For this review, take the finished solid that the model builds, in its own axes (mm). A direction names the side the tool comes from. Give positions to 0.01 mm unless a question says otherwise; leave off trailing zeros. Order: outer loops, then holes, each group sorted by start corner. A loop starts at its lowest first (then second) coordinate and runs counter-clockwise, first axis right, second up.
from build123d import *

# Parameters (mm, degrees)
CHAMFER1_SIZE = 1.25


with BuildPart() as part:
    # Sketch1 → Revolve1 (revolve)
    with BuildSketch(Plane(origin=(0, 0, 0), x_dir=(0, 0, -1), z_dir=(1, 0, 0))):
        with BuildLine():
            Line((0, 0), (0, 85.55))
            Line((0, 85.55), (3.18, 85.55))
            Line((3.18, 85.55), (3.18, 15.100044805))
            ThreePointArc((3.18, 15.100044805), (10.945145292, 4.426569715), (24.13, 3.81))
            Line((24.13, 3.81), (26.67, 1.27))
            Line((26.67, 1.27), (26.67, 0))
            Line((26.67, 0), (0, 0))
        make_face()
    revolve(axis=Axis((0, 0, 0), (0, 1, 0)))

    # Chamfer1
    chamfer1_edges = [part.edges().sort_by_distance(p)[0] for p in [
        (0, 85.55, 3.18),
    ]]
    chamfer(chamfer1_edges, length=CHAMFER1_SIZE)


solid = part.part
1) We need section A-A on z = 0. Give the boundary of the cut face in (x, y), then the cut area to 3 significant figures.
Answer sheet:
outline: (-26.67, 0) - (26.67, 0) - (26.67, 1.27) - (24.13, 3.81) arc R15.25 cw to (3.18, 15.1) - (3.18, 84.3) - (1.93, 85.55) - (-1.93, 85.55) - (-3.18, 84.3) - (-3.18, 15.1) arc R15.25 cw to (-24.13, 3.81) - (-26.67, 1.27) - close
area: 762 mm2
2) Tool access review of faces 1 (the face through (3.1, 49.2, 0.7)), 2 (the face through (0, 85.55, 0)): name each direction out of +Z, -Z, +X, -X, +Y, -Y from which nothing blocks a thin tool from reaching the whole face with its end or side.
Answer sheet:
face 1: +Y
face 2: +Z, -Z, +X, -X, +Y
3) We need section C-C on y = 63.5. Give the boundary of the cut face in (x, z).
Answer sheet:
outline: circle Ø6.36 at (0, 0)
4) To check wall thickness, follow line 1 (Y direction, x = 16, z = -7); line 2 (X direction, y = 5, z = 6); line 3 (Y direction, x = 7.5, z = 1). State the ranges of each line that lie inside material, in increasing order.
Answer sheet:
line 1: y = 0 to 2.62
line 2: x = -7.96 to 7.96
line 3: y = 0 to 6.9
5) We need section B-B on x = 0. Give the boundary of the cut face in (y, z).
Answer sheet:
outline: (0, -26.67) - (1.27, -26.67) - (3.81, -24.13) arc R15.25 cw to (15.1, -3.18) - (84.3, -3.18) - (85.55, -1.93) - (85.55, 1.93) - (84.3, 3.18) - (15.1, 3.18) arc R15.25 cw to (3.81, 24.13) - (1.27, 26.67) - (0, 26.67) - close
6) Clearance check with flat-ended pins moving along their axes: pin 1 (6 mm diameter, centred on y = 56.5, z = 3.5, fed in from -X); pin 2 (1.5 mm diameter, centred on x = 1, z = 16, fed in from +Y); pin 3 (1 mm diameter, centred on x = 14.5, z = -2.5, fed in from +Y); pin 4 (12 mm diameter, centred on x = 15, y = 15.5, fed in from +Z). State where each tip first meets the part, or that it passes through.
Answer sheet:
pin 1: stops at x = -3.14
pin 2: stops at y = 2.88
pin 3: stops at y = 3.13
pin 4: passes through
